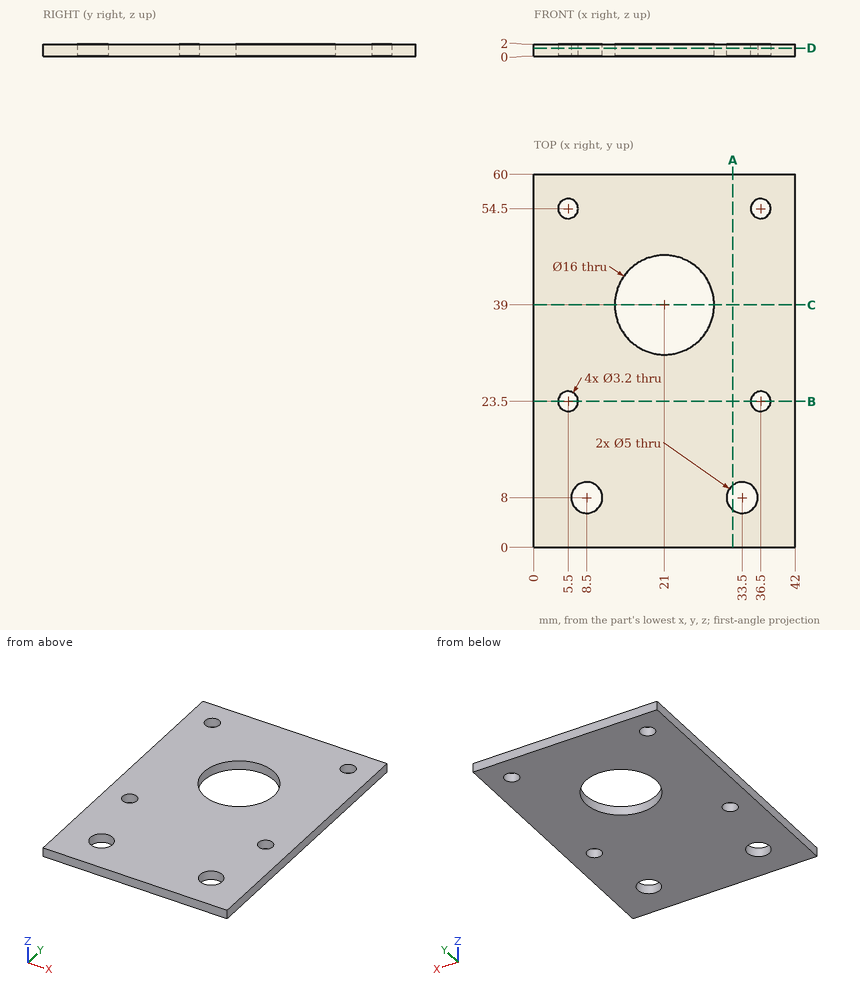
Design review of the part shown in the three views and the two pictorial views. Dimensions are in mm from the part's minimum x, y and z. Give positions to 0.01 mm unless a question says otherwise; leave off trailing zeros. Write each loop counter-clockwise with the first axis right and the second up, starting at its lowest first coordinate (ties: lowest second). Pieces come first, ordered by that corner, then holes. Notation, with made-up numbers: (-7, 56.5) -> (13, 56.5) arc R17 ccw to (13, 89.5) -> close; hole circle Ø1 at (50.5, 41). An arc over 180 degrees is marked (long way). Answer in a Markdown table with one row per item.
1) For L1, parallel to Y at x = 5.5, z = 0.65; L2, parallel to Y at x = 37, z = 0.7; L3, parallel to X at y = 54, z = 0.25, list the stretches that pass through material, from the lowest coordinate up. Write a range as [from, to].
Worked answers:
| item | result |
|---|---|
| L1 | [0, 21.9], [25.1, 52.9], [56.1, 60] |
| L2 | [0, 21.98], [25.02, 52.98], [56.02, 60] |
| L3 | [0, 3.98], [7.02, 34.98], [38.02, 42] |
2) Add section C-C on y = 39. State the section outline as (x, z) points, plus the area to 3 significant figures.
Worked answers:
| item | result |
|---|---|
| outline | (0, 0) -> (13, 0) -> (13, 2) -> (0, 2) -> close; (29, 0) -> (42, 0) -> (42, 2) -> (29, 2) -> close |
| area | 52.0 mm² |
3) Add section D-D on z = 1.35. State the section outline as (x, y) points, plus the area to 3 significant figures.
Worked answers:
| item | result |
|---|---|
| outline | (0, 0) -> (42, 0) -> (42, 60) -> (0, 60) -> close; hole circle Ø3.2 at (5.5, 23.5); hole circle Ø3.2 at (5.5, 54.5); hole circle Ø5 at (8.5, 8); hole circle Ø16 at (21, 39); hole circle Ø5 at (33.5, 8); hole circle Ø3.2 at (36.5, 23.5); hole circle Ø3.2 at (36.5, 54.5) |
| area | 2,250 mm² |
4) Clearance check with flat-ended pins moving along their axes: P1, Ø3, axis at x = 17, y = 12, coming from the -Z side; P2, Ø4.5, axis at x = 8.5, y = 8, coming from the -Z side. State where each tip first meets the part, or that it passes through.
Worked answers:
| item | result |
|---|---|
| P1 | z = 0 |
| P2 | through |
5) Add section A-A on x = 32. State the section outline as (y, z) points.
Worked answers:
| item | result |
|---|---|
| outline | (0, 0) -> (6, 0) -> (6, 2) -> (0, 2) -> close; (10, 0) -> (60, 0) -> (60, 2) -> (10, 2) -> close |
6) Add section B-B on y = 23.5. State the section outline as (x, z) points, plus the area to 3 significant figures.
Worked answers:
| item | result |
|---|---|
| outline | (0, 0) -> (3.9, 0) -> (3.9, 2) -> (0, 2) -> close; (7.1, 0) -> (34.9, 0) -> (34.9, 2) -> (7.1, 2) -> close; (38.1, 0) -> (42, 0) -> (42, 2) -> (38.1, 2) -> close |
| area | 71.2 mm² |
